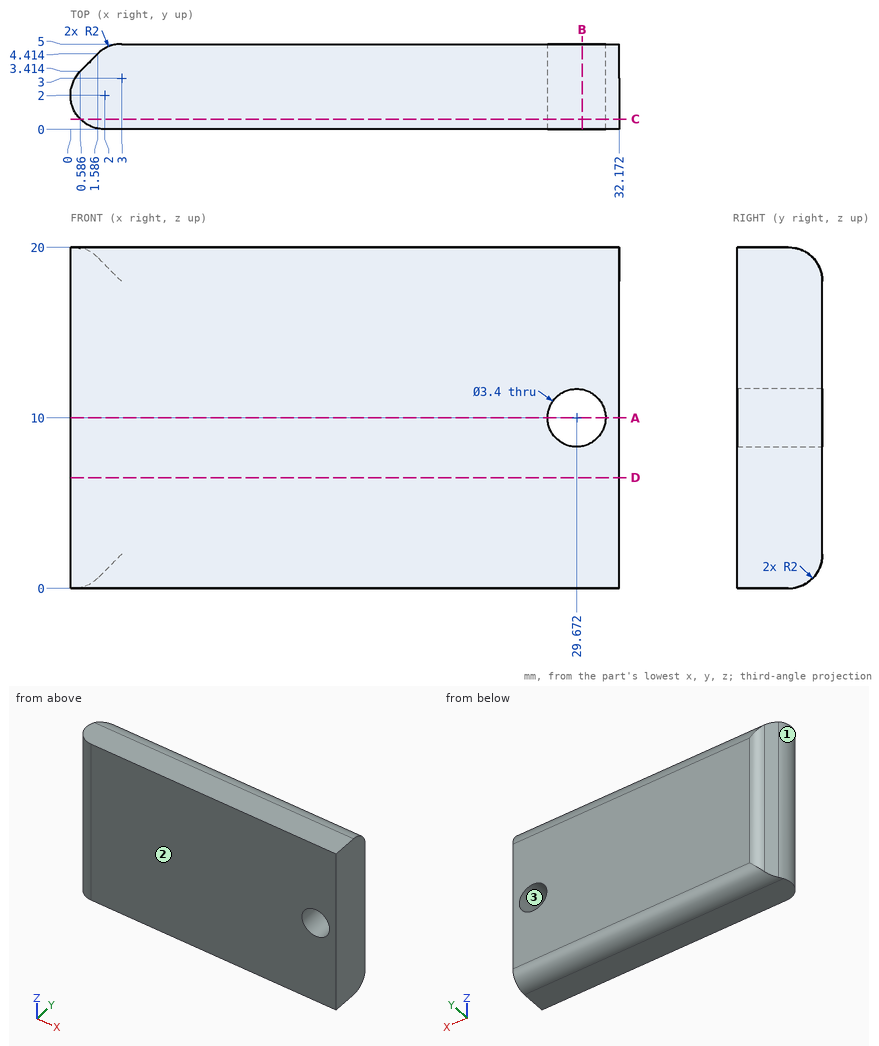
Verification items for this drawing (mm, ordinates from the low corner). Coordinates: 2 decimals unless noted, no trailing zeros. Write each loop counter-clockwise with the first axis right and the second up, starting at its lowest first coordinate (ties: lowest second). Pieces come first, ordered by that corner, then holes. Notation, with made-up numbers: (17.5, 28.25) -> (35.5, 28.25) arc R11 cw to (35.5, 45.25) -> close; hole circle Ø10 at (24.5, 29.25). An arc over 180 degrees is marked (long way). Use CSV: the item, a comma, the result in double quotes. Start each with the question number.
Item 1: Cross-section at B-B, the plane x = 30. Record the cut outline in (y, z).
Item 2: Cross-section at D-D, the plane z = 6.5. Record the cut outline in (x, y) (1 decimal).
Item 3: Depth check by flat-ended pin: pin 1 Ø1.5 at (y, z) = (3.5, 7.5) entering from -X (1 decimal). Enter the tip coordinate at first touch or a pass-through.
Item 4: Cross-section at A-A, the plane z = 10. Record the cut outline in (x, y) (1 decimal).
Item 5: Thickness scan on line 1 (X direction, y = 1.4, z = 10); line 2 (X direction, y = 3.6, z = 10); line 3 (X direction, y = 2.9, z = 7.5) (1 decimal). Record the ranges inside material, lowest first.
Item 6: Mould release check, pull along X, two halves, no side actions. Record for the marked faces 1, 2 and 3: released by +X, released by -X, zero draft, split by the parting line, or undercut.
Item 7: Cross-section at C-C, the plane y = 0.6. Record the cut outline in (x, z), plus the area to 3 significant figures.
Answers:
1,outline,"(0, 0) -> (3, 0) arc R2 ccw to (5, 2) -> (5, 8.33) -> (0, 8.33) -> close; (0, 11.67) -> (5, 11.67) -> (5, 18) arc R2 ccw to (3, 20) -> (0, 20) -> close"
2,outline,"(0.6, 3.4) arc R2 ccw to (2, 0) -> (32.2, 0) -> (32.2, 5) -> (3, 5) arc R2 ccw to (1.6, 4.4) -> close"
3,pin 1,"x = 0.1"
4,outline,"(0.6, 3.4) arc R2 ccw to (2, 0) -> (28, 0) -> (28, 5) -> (3, 5) arc R2 ccw to (1.6, 4.4) -> close; (31.4, 0) -> (32.2, 0) -> (32.2, 5) -> (31.4, 5) -> close"
5,line 1,"0.09 to 27.97, 31.37 to 32.17"
5,line 2,"0.77 to 27.97, 31.37 to 32.17"
5,line 3,"0.2 to 32.2"
6,face 1,"released by -X"
6,face 2,"zero draft"
6,face 3,"undercut"
7,outline,"(0.57, 0) -> (32.17, 0) -> (32.17, 20) -> (0.57, 20) -> close; hole circle Ø3.4 at (29.67, 10)"
7,area,"623 mm^2"
